CAD build for the part. Positions are in the model's coordinates, mm. Face numbers are marked on the shaded views. Give positions to 0.01 mm unless a question says otherwise; leave off trailing zeros. Loops run counter-clockwise (first coordinate to the right, second up) from the corner with the lowest first, then second, coordinate; pieces in that order, holes last.
Item 1: Saw through at B-B on x = 20.5. Give the cut face in (y, z).
Item 2: Drop a flat-ended pin along its axis: P1, Ø5, axis at x = 5, y = 14, coming from the -Z side. Give the stop position or say it passes through.
Item 3: Saw through at A-A on y = 8. Give the cut face in (x, z).
Item 4: Saw through at D-D on x = 0. Give the cut face in (y, z), plus the area to 3 significant figures.
Item 5: Saw through at C-C on y = 14. Give the cut face in (x, z), plus the area to 4 significant figures.
Item 6: Probe probe 1 along Y at (x, z) = (8.5, -0.45); probe 2 along Y at (x, z) = (3.75, -1.2); probe 3 along Y at (x, z) = (5, 1.15). List the from-to ranges inside material, lowest first.
Item 7: Mould opens along X. For the marked faces 1, 2, 3 and 4 say: released by +X, released by -X, zero draft, split by the parting line, or undercut.
from build123d import *

# Parameters (mm, degrees)
SKETCH_1_R      = 1.5
SKETCH_1_R_2    = 1.6
EXTRUDE_1_DEPTH = 1.5
CHAMFER_1_SIZE  = 1.5
FILLET_1_R      = 2.5
CHAMFER_2_SIZE  = 4


with BuildPart() as part:
    # 草图1 → 凸台-拉伸1 (new, symmetric)
    with BuildSketch(Plane.XY):
        with BuildLine():
            Line((-3.5, 17), (-3.5, -15))
            Line((-3.5, -15), (19.171710101, -25.152700357))
            ThreePointArc((19.171710101, -25.152700357), (22.789314225, -24.493379894), (23.476214014, -20.880910968))
            Line((23.476214014, -20.880910968), (13, 3))
            Line((13, 3), (13, 17))
            Line((13, 17), (-3.5, 17))
        make_face()
        Circle(SKETCH_1_R, mode=Mode.SUBTRACT)
        with Locations((10, -10)):
            Circle(SKETCH_1_R_2, mode=Mode.SUBTRACT)
        with Locations((20.5, -22.186533479)):
            Circle(SKETCH_1_R_2, mode=Mode.SUBTRACT)
        with Locations((0, 8)):
            Circle(SKETCH_1_R_2, mode=Mode.SUBTRACT)
        with Locations((10, 8)):
            Circle(SKETCH_1_R_2, mode=Mode.SUBTRACT)
        with Locations((5, 14)):
            Circle(SKETCH_1_R_2, mode=Mode.SUBTRACT)
    extrude(amount=EXTRUDE_1_DEPTH, both=True)

    # 倒角1
    # the kernel refuses this chamfer: 1.5 mm, written as the material it takes off along each edge
    with BuildSketch(Plane(origin=(10, -10, -1.5), x_dir=(1, 0, 0), z_dir=(0, -1, 0))) as chamfer_1_piece_1:
        Polygon((1.6, CHAMFER_1_SIZE), (1.6 + CHAMFER_1_SIZE, 0), (1.6, 0), align=None)
    revolve(axis=Axis((10, -10, -1.5), (0, 0, 1)), mode=Mode.SUBTRACT)
    with BuildSketch(Plane(origin=(20.5, -22.186533479, -1.5), x_dir=(1, 0, 0), z_dir=(0, -1, 0))) as chamfer_1_piece_2:
        Polygon((1.6, CHAMFER_1_SIZE), (1.6 + CHAMFER_1_SIZE, 0), (1.6, 0), align=None)
    revolve(axis=Axis((20.5, -22.186533479, -1.5), (0, 0, 1)), mode=Mode.SUBTRACT)
    with BuildSketch(Plane(origin=(0, 8, -1.5), x_dir=(1, 0, 0), z_dir=(0, -1, 0))) as chamfer_1_piece_3:
        Polygon((1.6, CHAMFER_1_SIZE), (1.6 + CHAMFER_1_SIZE, 0), (1.6, 0), align=None)
    revolve(axis=Axis((0, 8, -1.5), (0, 0, 1)), mode=Mode.SUBTRACT)
    with BuildSketch(Plane(origin=(10, 8, -1.5), x_dir=(1, 0, 0), z_dir=(0, -1, 0))) as chamfer_1_piece_4:
        Polygon((1.6, CHAMFER_1_SIZE), (1.6 + CHAMFER_1_SIZE, 0), (1.6, 0), align=None)
    revolve(axis=Axis((10, 8, -1.5), (0, 0, 1)), mode=Mode.SUBTRACT)
    with BuildSketch(Plane(origin=(5, 14, -1.5), x_dir=(1, 0, 0), z_dir=(0, -1, 0))) as chamfer_1_piece_5:
        Polygon((1.6, CHAMFER_1_SIZE), (1.6 + CHAMFER_1_SIZE, 0), (1.6, 0), align=None)
    revolve(axis=Axis((5, 14, -1.5), (0, 0, 1)), mode=Mode.SUBTRACT)

    # 圆角1
    fillet_1_edges = [part.edges().sort_by_distance(p)[0] for p in [
        (13, 3, 0),
        (-3.5, -15, 0),
    ]]
    fillet(fillet_1_edges, radius=FILLET_1_R)

    # 倒角2
    chamfer_2_edges = [part.edges().sort_by_distance(p)[0] for p in [
        (13, 17, 0),
        (-3.5, 17, 0),
    ]]
    chamfer(chamfer_2_edges, length=CHAMFER_2_SIZE)


solid = part.part
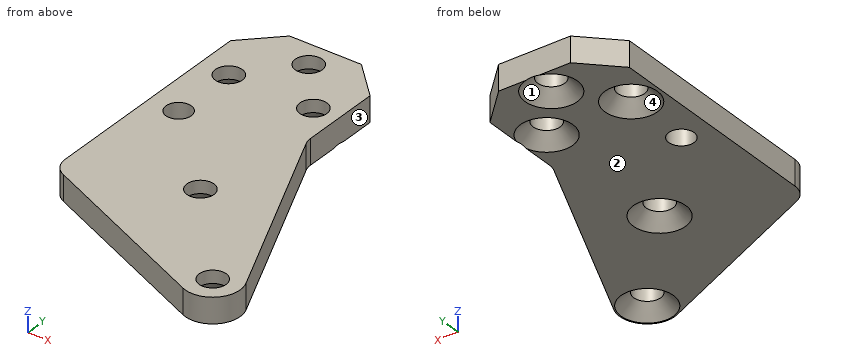
Results below:
1. outline: (-25.44, -1.5) - (-25.29, -1.5) - (-23.79, 0) - (-23.79, 1.5) - (-25.44, 1.5) - close; (-20.59, 0) - (-19.09, -1.5) - (-14.1, -1.5) - (-14.1, 1.5) - (-20.59, 1.5) - close
2. P1: stops at z = -0.9
3. outline: (-3.5, -1.5) - (-3.1, -1.5) - (-1.6, 0) - (-1.6, 1.5) - (-3.5, 1.5) - close; (1.6, 0) - (3.1, -1.5) - (6.9, -1.5) - (8.4, 0) - (8.4, 1.5) - (1.6, 1.5) - close; (11.6, 0) - (13, -1.4) - (13, 1.5) - (11.6, 1.5) - close
4. outline: (-16.57, -1.5) - (-1.5, -1.5) - (-1.5, 1.5) - (-16.57, 1.5) - close; (1.5, -1.5) - (4.9, -1.5) - (6.4, 0) - (6.4, 1.5) - (1.5, 1.5) - close; (9.6, 0) - (11.1, -1.5) - (16.5, -1.5) - (16.5, 1.5) - (9.6, 1.5) - close
4. area: 78.4 mm2
5. outline: (-2.5, -1.5) - (1.9, -1.5) - (3.4, 0) - (3.4, 1.5) - (-2.5, 1.5) - close; (6.6, 0) - (8.1, -1.5) - (12, -1.5) - (12, 1.5) - (6.6, 1.5) - close
5. area: 31.65 mm2
6. probe 1: y = -20.37 to -11.4, -8.6 to 6.6, 9.4 to 17
6. probe 2: y = -18.25 to 11.49, 16.51 to 17
6. probe 3: y = -18.81 to 12.4, 15.6 to 17
7. face 1: undercut
7. face 2: zero draft
7. face 3: released by +X
7. face 4: undercut
